Part model, mm, in its own coordinate system. A direction names the side the tool comes from. Give positions to 0.01 mm unless a question says otherwise; leave off trailing zeros. Write each loop counter-clockwise with the first axis right and the second up, starting at its lowest first coordinate (ties: lowest second). Pieces come first, ordered by that corner, then holes. Notation, with made-up numbers: M -13.5,8.5 L 18.5,8.5 A30 cw 18.5,35.5 Z; hole C -0.75,63.25 d3. An arc over 180 degrees is marked long. Write item = value, one per line. Start each with the question number.
from build123d import *

# Parameters (mm, degrees)
BOSS_EXTRUDE1_DEPTH = 15
SKETCH2_R           = 3
CUT_EXTRUDE1_DEPTH  = 30
SKETCH3_W           = 35
SKETCH3_H           = 10
CUT_EXTRUDE2_DEPTH  = 50.694064129
FILLET1_R           = 4
SKETCH4_R           = 6
CUT_EXTRUDE3_DEPTH  = 30
FILLET2_R           = 4
CHAMFER1_SIZE       = 3


with BuildPart() as part:
    # Sketch1 → Boss-Extrude1 (new, symmetric)
    with BuildSketch(Plane(origin=(0, 0, 0), x_dir=(1, 0, 0), z_dir=(0, 1, 0))):
        with BuildLine():
            ThreePointArc((-28.253318389, -18), (-31.709094157, -10.806634433), (-33.365401241, -3))
            Line((-33.365401241, -3), (-33.5, -3))
            Line((-33.5, -3), (-33.5, -18))
            Line((-33.5, -18), (-28.253318389, -18))
        make_face()
        with BuildLine():
            Line((33.365401241, -3), (23.307724042, -3))
            ThreePointArc((23.307724042, -3), (0, -23.5), (-23.307724042, -3))
            Line((-23.307724042, -3), (-33.365401241, -3))
            ThreePointArc((-33.365401241, -3), (-31.709094157, -10.806634433), (-28.253318389, -18))
            ThreePointArc((-28.253318389, -18), (0, -33.5), (28.253318389, -18))
            ThreePointArc((28.253318389, -18), (31.709094157, -10.806634433), (33.365401241, -3))
        make_face()
        with BuildLine():
            Line((33.5, -3), (33.365401241, -3))
            ThreePointArc((33.365401241, -3), (31.709094157, -10.806634433), (28.253318389, -18))
            Line((28.253318389, -18), (33.5, -18))
            Line((33.5, -18), (33.5, -3))
        make_face()
    extrude(amount=BOSS_EXTRUDE1_DEPTH, both=True)

    # Sketch2 → Cut-Extrude1 (cut)
    with BuildSketch(Plane.XY):
        with Locations(Location((29, -9, 0), (0, 0, 180))):
            Circle(SKETCH2_R)
        with Locations(Location((29, 9, 0), (0, 0, 180))):
            Circle(SKETCH2_R)
        with Locations(Location((-29, 9, 0), (0, 0, 284.412066788))):
            Circle(SKETCH2_R)
        with Locations(Location((-29, -9, 0), (0, 0, 75.587933212))):
            Circle(SKETCH2_R)
    extrude(amount=CUT_EXTRUDE1_DEPTH, mode=Mode.SUBTRACT)

    # Sketch3 → Cut-Extrude2 (cut, through all)
    with BuildSketch(Plane.XY):
        Rectangle(SKETCH3_W, SKETCH3_H)
    extrude(amount=CUT_EXTRUDE2_DEPTH, mode=Mode.SUBTRACT)

    # Fillet1
    fillet1_edges = [part.edges().sort_by_distance(p)[0] for p in [
        (17.5, -5, 22.125050428),
        (17.5, 5, 22.125050428),
        (-17.5, 5, 22.125050428),
        (-17.5, -5, 22.125050428),
    ]]
    fillet(fillet1_edges, radius=FILLET1_R)

    # Sketch4 → Cut-Extrude3 (cut)
    with BuildSketch(Plane.XY.offset(18)):
        with Locations((29, 9)):
            Circle(SKETCH4_R)
        with Locations((29, -9)):
            Circle(SKETCH4_R)
        with Locations((-29, -9)):
            Circle(SKETCH4_R)
        with Locations((-29, 9)):
            Circle(SKETCH4_R)
    extrude(amount=CUT_EXTRUDE3_DEPTH, mode=Mode.SUBTRACT)

    # Fillet2
    # the kernel refuses this fillet: 4 mm, written as the material it adds along each edge
    with BuildSketch(Plane(origin=(28.253318389, 8.334769634, 18), x_dir=(1, 0, 0), z_dir=(0, -1, 0))) as fillet2_piece_1_section:
        with BuildLine():
            CenterArc((2.115250889, 4), FILLET2_R, 215.920819838, 54.079180162)
            ThreePointArc((-1.124063167, 1.653333333), (-0.549695111, 0.835053949), (0, 0))
            Line((0, 0), (2.115250889, 0))
        make_face()
    fillet2_piece_1 = extrude(amount=16.669539268, mode=Mode.PRIVATE)
    fillet2_piece_1 = fillet2_piece_1 - Plane(origin=(29, 9, 18.362807828), x_dir=(1, 0, 0), z_dir=(0, 0, -1)) * Cylinder(6, 42, mode=Mode.PRIVATE)
    fillet2_piece_1 = fillet2_piece_1 - Plane(origin=(29, -9, 18.362807828), x_dir=(1, 0, 0), z_dir=(0, 0, -1)) * Cylinder(6, 42, mode=Mode.PRIVATE)
    add(fillet2_piece_1)
    with BuildSketch(Plane(origin=(-28.253318389, -8.334769634, 18), x_dir=(-1, 0, 0), z_dir=(0, 1, 0))) as fillet2_piece_2_section:
        with BuildLine():
            CenterArc((2.115250889, 4), FILLET2_R, 215.920819838, 54.079180162)
            ThreePointArc((-1.124063167, 1.653333333), (-0.549695111, 0.835053949), (0, 0))
            Line((0, 0), (2.115250889, 0))
        make_face()
    fillet2_piece_2 = extrude(amount=16.669539268, mode=Mode.PRIVATE)
    fillet2_piece_2 = fillet2_piece_2 - Plane(origin=(-29, -9, 18.362807828), x_dir=(1, 0, 0), z_dir=(0, 0, -1)) * Cylinder(6, 42, mode=Mode.PRIVATE)
    fillet2_piece_2 = fillet2_piece_2 - Plane(origin=(-29, 9, 18.362807828), x_dir=(1, 0, 0), z_dir=(0, 0, -1)) * Cylinder(6, 42, mode=Mode.PRIVATE)
    add(fillet2_piece_2)

    # Chamfer1
    # the kernel refuses this chamfer: 3 mm, written as the material it takes off along each edge
    with BuildSketch(Plane(origin=(33.5, -15, 25.715048964), x_dir=(-0.9996219169112968, -0.02749587661058619, 0), z_dir=(0, 0, -1)), Plane(origin=(-33.5, 15, -4.715048964), x_dir=(-0.02749587661058678, -0.9996219169112968, 0), z_dir=(0, 0, 1))) as chamfer1_piece_1:
        Polygon((CHAMFER1_SIZE * 0.999621916911, CHAMFER1_SIZE * 0.0274958766106), (-CHAMFER1_SIZE * 0.0274958766106, CHAMFER1_SIZE * 0.999621916911), (0, 0), align=None)
    extrude(amount=30.430097928, mode=Mode.SUBTRACT)
    with BuildSketch(Plane(origin=(-33.5, 22.715048964, 3), x_dir=(-0.02749587661058677, 0, 0.9996219169112968), z_dir=(0, -1, 0)), Plane(origin=(33.5, -22.715048964, 3), x_dir=(0.027495876610586757, 0, 0.9996219169112968), z_dir=(0, 1, 0))) as chamfer1_piece_2:
        Polygon((CHAMFER1_SIZE * 0.999621916911, -CHAMFER1_SIZE * 0.0274958766106), (-CHAMFER1_SIZE * 0.0274958766106, -CHAMFER1_SIZE * 0.999621916911), (0, 0), align=None)
    extrude(amount=45.430097928, mode=Mode.SUBTRACT)
    with BuildSketch(Plane(origin=(33.5, 15, 25.715048964), x_dir=(-0.9996219169112968, 0.02749587661058619, 0), z_dir=(0, 0, -1)), Plane(origin=(-33.5, -15, -4.715048964), x_dir=(-0.02749587661058678, 0.9996219169112968, 0), z_dir=(0, 0, 1))) as chamfer1_piece_3:
        Polygon((CHAMFER1_SIZE * 0.999621916911, -CHAMFER1_SIZE * 0.0274958766106), (-CHAMFER1_SIZE * 0.0274958766106, -CHAMFER1_SIZE * 0.999621916911), (0, 0), align=None)
    extrude(amount=30.430097928, mode=Mode.SUBTRACT)


solid = part.part
Q1. Probe line 1 along Y through (x, z) = (-29, 6); line 2 along X through (y, z) = (11.5, 8.5); line 3 along X through (y, z) = (9, 12). List the from-to ranges inside material, lowest first.
Q2. Drop flat-ended pins along their axis: P1, Ø9.5, axis at x = 29, y = -9, coming from the +Z side; P2, Ø6, axis at x = 17, y = -9, coming from the -Z side; P3, Ø5, axis at x = -8.5, y = 11.5, coming from the +Z side. Give the stop position or say it passes through.
Q3. Slice it at C-C (z = 11). Give the cut face in (x, y).
Q4. Slice it at B-B (x = 12). Give the cut face in (y, z), and give its area (3 significant figures).
Q5. Slice it at D-D (x = 29). Give the cut face in (y, z), and give its area (3 significant figures).
Q6. Tool access for faces 4 (the face through (26, 0, 3)), 5 (the face through (-17.5, 0, 22)): list every direction of +Z, -Z, +X, -X, +Y, -Y with a clear straight run to the whole face (end or side of a thin tool).
Q7. Two-plate mould, pull along Y, no slides. Class faces 1 (the face through (-26.08, -8.32, 10.39)), 2 (the face through (0, -15, 25)), 3 (the face through (-33.5, 0, 12)): +Y half, -Y half, draft (parallel to the pull), parting line (faces both ways), or undercut.
Q8. Slice it at A-A (z = 16.5). Give the cut face in (x, y), and give its area (3 significant figures).
Working result:
q1.line_1 = -15 to -12, -6 to 6, 12 to 15
q1.line_2 = -33.5 to -30.66, -27.34 to -21.91, 21.91 to 27.34, 30.66 to 33.5
q1.line_3 = -33.5 to -32, -26 to -20.21, 20.21 to 26, 32 to 33.5
q2.P1 = 18
q2.P2 = 12.34
q2.P3 = 32.96
q3.outline = M -33.5,-12 L -30.5,-15 L -20.77,-15 L -20.77,15 L -30.5,15 L -33.5,12 Z; M 20.77,-15 L 30.5,-15 L 33.5,-12 L 33.5,12 L 30.5,15 L 20.77,15 Z; hole C -29,-9 d6; hole C -29,9 d6; hole C 29,-9 d6; hole C 29,9 d6
q4.outline = M -15,20.21 L -5,20.21 L -5,31.28 L -15,31.28 Z; M 5,20.21 L 15,20.21 L 15,31.28 L 5,31.28 Z
q4.area = 221 mm2
q5.outline = M -15,3 L -12,3 L -12,18 L -15,18 Z; M -6,3 L 6,3 L 6,18 L 3,18 L 3,18.24 L -3,18.24 L -3,18 L -6,18 Z; M 12,3 L 15,3 L 15,18 L 12,18 Z
q5.area = 271 mm2
q6.face_4 = -Z, +X, -X, +Y, -Y
q6.face_5 = +Z, -Z
q7.face_1 = undercut
q7.face_2 = -Y half
q7.face_3 = draft
q8.outline = M -33.5,-12 L -30.5,-15 L -16.73,-15 L -16.73,-3.36 A4 cw -17.5,-1 L -17.5,1 A4 cw -16.73,3.36 L -16.73,15 L -30.5,15 L -33.5,12 Z; M 16.73,-15 L 30.5,-15 L 33.5,-12 L 33.5,12 L 30.5,15 L 16.73,15 L 16.73,3.36 A4 cw 17.5,1 L 17.5,-1 A4 cw 16.73,-3.36 Z; hole C -29,-9 d6; hole C -29,9 d6; hole C 29,-9 d6; hole C 29,9 d6
q8.area = 867 mm2
